from build123d import *

# Parameters (mm, degrees)
F0_R     = 12.7
F1_DEPTH = 279.4
F3_DEPTH = 2.54
F4_DEPTH = 19.05


with BuildPart() as f1:
    # F0 (on Front) → F1 (new body)
    with BuildSketch(Plane.XZ):
        Circle(F0_R)
    extrude(amount=F1_DEPTH)

    # F2 (on face) → F3 (cut)
    with BuildSketch(Plane.XZ.offset(279.4)):
        with BuildLine():
            ThreePointArc((-5.5537875001, -3.0786270322), (-6.3227011551, -0.5881752316), (-6.026359286, 2.0013729678))
            Line((-6.026359286, 2.0013729678), (-12.5413119826, 2.0013729678))
            ThreePointArc((-12.5413119826, 2.0013729678), (-12.6880955617, -0.549755415), (-12.3212034963, -3.0786270322))
            Line((-12.3212034963, -3.0786270322), (-5.5537875001, -3.0786270322))
        make_face()
        with BuildLine():
            ThreePointArc((-2.54, 5.8198711326), (0, 6.35), (2.54, 5.8198711326))
            Line((2.54, 5.8198711326), (2.54, 12.4434078933))
            ThreePointArc((2.54, 12.4434078933), (0, 12.7), (-2.54, 12.4434078933))
            Line((-2.54, 12.4434078933), (-2.54, 5.8198711326))
        make_face()
        with BuildLine():
            ThreePointArc((6.026359286, 2.0013729678), (6.2685676779, 1.0136859805), (6.35, 0))
            ThreePointArc((6.35, 0), (6.1477252145, -1.589960593), (5.5537875001, -3.0786270322))
            Line((5.5537875001, -3.0786270322), (12.3212034963, -3.0786270322))
            ThreePointArc((12.3212034963, -3.0786270322), (12.6049451487, -1.5509215966), (12.7, 0))
            ThreePointArc((12.7, 0), (12.660265838, 1.0038271319), (12.5413119826, 2.0013729678))
            Line((12.5413119826, 2.0013729678), (6.026359286, 2.0013729678))
        make_face()
        with BuildLine():
            Line((2.54, -12.4434078933), (2.54, -5.8198711326))
            ThreePointArc((2.54, -5.8198711326), (0, -6.35), (-2.54, -5.8198711326))
            Line((-2.54, -5.8198711326), (-2.54, -12.4434078933))
            ThreePointArc((-2.54, -12.4434078933), (0, -12.7), (2.54, -12.4434078933))
        make_face()
    extrude(amount=-F3_DEPTH, mode=Mode.SUBTRACT)

    # F2 (on face) → F4 (cut)
    with BuildSketch(Plane.XZ.offset(279.4)):
        with BuildLine():
            ThreePointArc((5.5537875001, -3.0786270322), (6.1477252145, -1.589960593), (6.35, 0))
            ThreePointArc((6.35, 0), (6.2685676779, 1.0136859805), (6.026359286, 2.0013729678))
            ThreePointArc((6.026359286, 2.0013729678), (4.689441322, 4.2815464598), (2.54, 5.8198711326))
            ThreePointArc((2.54, 5.8198711326), (0, 6.35), (-2.54, 5.8198711326))
            ThreePointArc((-2.54, 5.8198711326), (-4.689441322, 4.2815464598), (-6.026359286, 2.0013729678))
            ThreePointArc((-6.026359286, 2.0013729678), (-6.3227011551, -0.5881752316), (-5.5537875001, -3.0786270322))
            ThreePointArc((-5.5537875001, -3.0786270322), (-4.2726986588, -4.6975042492), (-2.54, -5.8198711326))
            ThreePointArc((-2.54, -5.8198711326), (0, -6.35), (2.54, -5.8198711326))
            ThreePointArc((2.54, -5.8198711326), (4.2726986588, -4.6975042492), (5.5537875001, -3.0786270322))
        make_face()
    extrude(amount=-F4_DEPTH, mode=Mode.SUBTRACT)


solid = f1.part
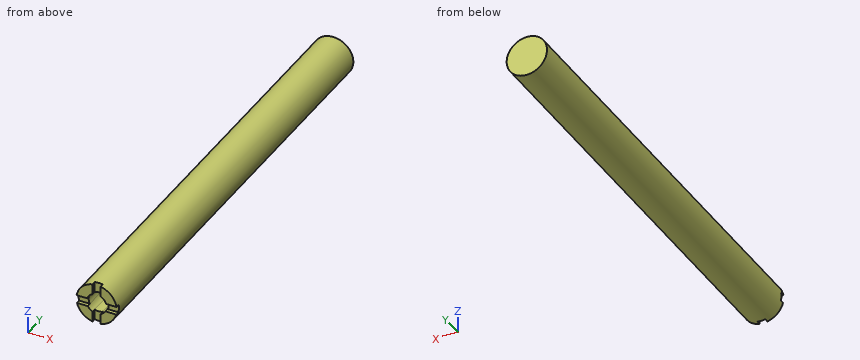
Verification items for the finished model (mm, model axes). Give positions to 0.01 mm unless a question says otherwise; leave off trailing zeros. Write each loop counter-clockwise with the first axis right and the second up, starting at its lowest first coordinate (ties: lowest second). Pieces come first, ordered by that corner, then holes. Notation, with made-up numbers: (88, -7) - (129, -7) arc R23 cw to (129, 17) - close; hole circle Ø1 at (36, -3). An arc over 180 degrees is marked (long way). Answer as CSV lines item,"result". Start each with the question number.
1. Sectioned sample at A-A (x = 0). Record the boundary of the cut face in (y, z).
2. Thickness scan on line 1 (X direction, y = -51.5, z = -1.75); line 2 (Y direction, x = 2.5, z = 7.25); line 3 (Z direction, x = 11, y = -51.5). Record the ranges inside material, lowest first.
3. Sectioned sample at B-B (y = -256). Record the boundary of the cut face in (x, z), then the cut area to 3 significant figures.
4. Depth check by flat-ended pin: pin 1 (2.5 mm diameter, centred on x = -1, z = 8.5, fed in from -Y); pin 2 (1.3 mm diameter, centred on y = -277.5, z = -10.5, fed in from -X); pin 3 (2 mm diameter, centred on x = -7.5, y = -278, fed in from +Z). Enter the tip coordinate at first touch or a pass-through.
Derived:
1,outline,"(-276.86, -12.7) - (0, -12.7) - (0, 12.7) - (-276.86, 12.7) - (-276.86, 6.35) - (-260.35, 6.35) - (-260.35, -6.35) - (-276.86, -6.35) - close"
2,line 1,"-12.58 to 12.58"
2,line 2,"-276.86 to 0"
2,line 3,"-6.35 to 6.35"
3,outline,"circle Ø25.4 at (0, 0)"
3,area,"507 mm²"
4,pin 1,"y = -276.86"
4,pin 2,"x = -8.02"
4,pin 3,"z = 10.91"
